from build123d import *

# Parameters (mm, degrees)
F0_R     = 32.5
F1_DEPTH = 1
F0_R_2   = 30
F2_DEPTH = 0.5
F3_DEPTH = 4
F3_TAPER = -15


with BuildPart() as f1:
    # F0 (on Top) → F1 (new body)
    with BuildSketch(Plane.XY):
        with BuildLine():
            Line((-38, -35), (38, -35))
            Line((38, -35), (38, -29.5))
            ThreePointArc((38, -29.5), (36.9393398282, -26.9393398282), (39.5, -28))
            Line((39.5, -28), (45, -28))
            Line((45, -28), (45, 28))
            Line((45, 28), (39.5, 28))
            ThreePointArc((39.5, 28), (36.9393398282, 26.9393398282), (38, 29.5))
            Line((38, 29.5), (38, 35))
            Line((38, 35), (-38, 35))
            Line((-38, 35), (-38, 29.5))
            ThreePointArc((-38, 29.5), (-36.9393398282, 29.0606601718), (-36.5, 28))
            ThreePointArc((-36.5, 28), (-38, 26.5), (-39.5, 28))
            Line((-39.5, 28), (-45, 28))
            Line((-45, 28), (-45, -28))
            Line((-45, -28), (-39.5, -28))
            ThreePointArc((-39.5, -28), (-38, -26.5), (-36.5, -28))
            ThreePointArc((-36.5, -28), (-36.9393398282, -29.0606601718), (-38, -29.5))
            Line((-38, -29.5), (-38, -35))
        make_face()
        Circle(F0_R, mode=Mode.SUBTRACT)
        with BuildLine():
            Line((-45, 35), (-45, 28))
            Line((-45, 28), (-39.5, 28))
            ThreePointArc((-39.5, 28), (-39.0606601718, 29.0606601718), (-38, 29.5))
            Line((-38, 29.5), (-38, 35))
            Line((-38, 35), (-45, 35))
        make_face()
        with BuildLine():
            Line((39.5, 28), (45, 28))
            Line((45, 28), (45, 35))
            Line((45, 35), (38, 35))
            Line((38, 35), (38, 29.5))
            ThreePointArc((38, 29.5), (39.0606601718, 29.0606601718), (39.5, 28))
        make_face()
        with BuildLine():
            Line((38, -35), (45, -35))
            Line((45, -35), (45, -28))
            Line((45, -28), (39.5, -28))
            ThreePointArc((39.5, -28), (39.0606601718, -29.0606601718), (38, -29.5))
            Line((38, -29.5), (38, -35))
        make_face()
        with BuildLine():
            Line((-45, -35), (-38, -35))
            Line((-38, -35), (-38, -29.5))
            ThreePointArc((-38, -29.5), (-39.0606601718, -29.0606601718), (-39.5, -28))
            Line((-39.5, -28), (-45, -28))
            Line((-45, -28), (-45, -35))
        make_face()
    extrude(amount=F1_DEPTH)



with BuildPart() as f2:
    # F0 (on Top) → F2 (new body)
    with BuildSketch(Plane.XY):
        Circle(F0_R_2)
    extrude(amount=F2_DEPTH)


with BuildPart() as f1_1:
    add(f1.part)

    add(f2.part)  # F3 merges F2
    # F0 (on Top) → F3 (join)
    with BuildSketch(Plane.XY):
        Circle(F0_R)
        Circle(F0_R_2, mode=Mode.SUBTRACT)
    extrude(amount=F3_DEPTH, taper=F3_TAPER)


solid = f1_1.part
Can you work these out from the model? Positions are in its coordinate system, mm. A direction names the side the tool comes from. Coordinates: 2 decimals unless noted, no trailing zeros. Loops run counter-clockwise (first coordinate to the right, second up) from the corner with the lowest first, then second, coordinate; pieces in that order, holes last. Notation, with made-up numbers: M 77,57 L 117,57 A21 ccw 117,63 Z; hole C 83,7 d2. An arc over 180 degrees is marked long. Return JSON: item names as keys, results as strings. Group by question number.
Item 1: Imagine slicing it at B-B (z = 1.8). Please give me the cut outline in (x, y).
Item 2: I'm going to push flat-ended pins straight in: pin 1 Ø1.8 at (x, y) = (38, 28) entering from -Z; pin 2 Ø3 at (x, y) = (-27, -28) entering from -Z; pin 3 Ø5 at (x, y) = (38, -28) entering from +Z; pin 4 Ø1.5 at (x, z) = (-27.5, 2) entering from -Y. Where does each tip first touch, or does it pass through?
Item 3: Imagine slicing it at A-A (x = 0). Please give me the cut outline in (y, z), and give its area (3 significant figures).
Item 4: On a 3-axis mill with a long thin cutter (end or side, diameter ignored), from which of +Z, -Z, +X, -X, +Y, -Y can I reach the whole of each face in a straight line? I mean faces 3 (the conical face through (31.303, 9.858, 1.188)), 4 (the flat face through (15, 25, 4)). Say none if no direction works.
Item 5: Thinking about a two-plate mould opening in X: for faces 1 (the conical face through (27.636, -8.703, 3.83)), 2 (the flat face through (-1, 0, 0)), which applies, released by +X, released by -X, zero draft, split by the parting line, or undercut?
Item 6: Imagine slicing it at C-C (x = 35.5). Please give me the cut outline in (y, z), and give its area (3 significant figures).
Item 7: If I drill on L1, parallel to Y at x = 38, z = 0.35; L2, parallel to Z at x = -26, y = -28.5; L3, parallel to Z at x = -0.5, y = -15.5, over which ranges is the centre line in solid material (lowest first)? Write a range as from..to.
Verdict:
{
 "1": {"outline": "C 0,0 d65.96; hole C 0,0 d59.04"},
 "2": {"pin 1": "passes through", "pin 2": "stops at z = 0", "pin 3": "stops at z = 1", "pin 4": "stops at y = -19.44"},
 "3": {"outline": "M -35,0 L 35,0 L 35,1 L 32.77,1 L 33.57,4 L 28.93,4 L 29.87,0.5 L -29.87,0.5 L -28.93,4 L -33.57,4 L -32.77,1 L -35,1 Z", "area": "63.2 mm^2"},
 "4": {"face 3": "none", "face 4": "+Z, +X, -X, +Y, -Y"},
 "5": {"face 1": "undercut", "face 2": "zero draft"},
 "6": {"outline": "M -35,0 L 35,0 L 35,1 L -35,1 Z", "area": "70.0 mm^2"},
 "7": {"L1": "y = -35..-29.5, -26.5..26.5, 29.5..35", "L2": "z = 0..1", "L3": "z = 0..0.5"}
}
